```python
from build123d import *

# Parameters (mm, degrees)
F0_W     = 105
F0_H     = 60
F1_DEPTH = 10
F2_R     = 2.5


with BuildPart() as f1:
    # F0 (on Front) → F1 (new body, symmetric)
    with BuildSketch(Plane.XZ):
        Rectangle(F0_W, F0_H)
        with BuildLine():
            ThreePointArc((-17.499497, 0.086824), (-17.499623, 0.043411), (-17.5, 0))
            ThreePointArc((-17.5, 0), (-32.499372, 0.130237), (-17.499497, 0.086824))
        make_face(mode=Mode.SUBTRACT)
        with BuildLine():
            ThreePointArc((-7.5, 0), (0, 7.5), (7.5, 0))
            ThreePointArc((7.5, 0), (0, -7.5), (-7.5, 0))
        make_face(mode=Mode.SUBTRACT)
        with BuildLine():
            ThreePointArc((32.492652, 0.33191), (25.158648, -7.166253), (17.5, 0))
            ThreePointArc((17.5, 0), (24.826656, 7.830073), (32.492652, 0.33191))
        make_face(mode=Mode.SUBTRACT)
    extrude(amount=F1_DEPTH, both=True)

    # F2
    f2_edges = [f1.edges().sort_by_distance(p)[0] for p in [
        (0, -10, 30),
        (-52.5, -10, 0),
        (0, -10, -30),
        (52.5, -10, 0),
    ]]
    fillet(f2_edges, radius=F2_R)


solid = f1.part
```
Geometry: final body of the model. Coordinates: model frame, mm. Round coordinates to 2 decimals unless told otherwise and drop trailing zeros. Order: outer loops, then holes, each group sorted by start corner. A loop starts at its lowest first (then second) coordinate and runs counter-clockwise, first axis right, second up. Notation, with made-up numbers: (9.5, 37.5) -> (15.5, 37.5) arc R26 ccw to (15.5, 75.5) -> close; hole circle Ø1 at (36.5, 23.5). An arc over 180 degrees is marked (long way). Use one line per item in the form item = value. Start each with the question number.
1. Draft query along X for faces 1 (the face through (-1.63, -0.14, 7.32)), 2 (the face through (-52.5, 1, 0)), 3 (the face through (0.735, -9.287, -29.248)). Return one class per face: pulls with the +X half, pulls with the -X half, needs draft (parallel to the pull), parting line crosses it, or undercut.
2. Cut plane C-C (y = -8.5). Return the cut outline in (x, z).
3. Cut plane B-B (y = -2.25). Return the cut outline in (x, z).
4. Line query: probe 1 along Z at (x, y) = (0, 4.75); probe 2 along X at (y, z) = (-0.25, 6.5); probe 3 along X at (y, z) = (-7.75, 17). Output: solid intervals per line, ascending.
5. Cut plane A-A (x = -1.5). Return the cut outline in (y, z), then the cut area to 3 significant figures.
6. Pin query (flat end, axial travel): pin 1 Ø13.5 at (x, z) = (0, 0) entering from +Y (3 decimals). Return the tip coordinate at first contact, or that it passes through.
Solution:
q1.face_1 = undercut
q1.face_2 = pulls with the -X half
q1.face_3 = needs draft
q2.outline = (-52.29, -29.79) -> (52.29, -29.79) -> (52.29, 29.79) -> (-52.29, 29.79) -> close; hole (-17.5, 0) arc R7.51 ccw to (-17.5, 0.09) arc R7.5 ccw (long way) to start; hole circle Ø15 at (0, 0); hole circle Ø15 at (24.99, 0.33)
q3.outline = (-52.5, -30) -> (52.5, -30) -> (52.5, 30) -> (-52.5, 30) -> close; hole (-17.5, 0) arc R7.51 ccw to (-17.5, 0.09) arc R7.5 ccw (long way) to start; hole circle Ø15 at (0, 0); hole circle Ø15 at (24.99, 0.33)
q4.probe_1 = -30 to -7.5, 7.5 to 30
q4.probe_2 = -52.5 to -28.89, -21.11 to -3.74, 3.74 to 20.73, 29.26 to 52.5
q4.probe_3 = -52.49 to 52.49
q5.outline = (-10, -27.5) arc R2.5 ccw to (-7.5, -30) -> (10, -30) -> (10, -7.35) -> (-10, -7.35) -> close; (-10, 7.35) -> (10, 7.35) -> (10, 30) -> (-7.5, 30) arc R2.5 ccw to (-10, 27.5) -> close
q5.area = 903 mm^2
q6.pin_1 = through
